```python
from build123d import *

# Parameters (mm, degrees)
F0_W      = 29.9564684167
F0_H      = 51
F0_R      = 5.425
F0_R_2    = 5.95
F1_DEPTH  = 25
F0_W_2    = 18.5217657917
F2_DEPTH  = 25
F0_R_3    = 3.415
F3_DEPTH  = 3.55
F4_R      = 2.34
F5_DEPTH  = 7.5
F7_START  = 14.1
F6_R      = 13
F7_DEPTH  = 10.9
F8_DEPTH  = 10.9
F9_R      = 2.5
F10_DEPTH = 5
F10_TAPER = 15
F11_R     = 5


with BuildPart() as f1:
    # F0 (on Top) → F1 (new body)
    with BuildSketch(Plane.XY):
        with Locations((0, -8)):
            Rectangle(F0_W, F0_H)
        with Locations((0, -25.365)):
            Circle(F0_R, mode=Mode.SUBTRACT)
        Circle(F0_R_2, mode=Mode.SUBTRACT)
    extrude(amount=F1_DEPTH)

    # F0 (on Top) → F2 (join)
    with BuildSketch(Plane.XY):
        with Locations((-24.2391171042, -8)):
            Rectangle(F0_W_2, F0_H)
        with Locations((-25.365, 0)):
            Circle(F0_R, mode=Mode.SUBTRACT)
        with Locations((24.2391171042, -8)):
            Rectangle(F0_W_2, F0_H)
        with Locations((25.365, 0)):
            Circle(F0_R, mode=Mode.SUBTRACT)
    extrude(amount=F2_DEPTH)

    # F0 (on Top) → F3 (join)
    with BuildSketch(Plane.XY):
        with Locations((-25.365, 0)):
            Circle(F0_R)
        with Locations((-25.365, 0)):
            Circle(F0_R_3, mode=Mode.SUBTRACT)
        with Locations((25.365, 0)):
            Circle(F0_R)
        with Locations((25.365, 0)):
            Circle(F0_R_3, mode=Mode.SUBTRACT)
        with Locations((0, -25.365)):
            Circle(F0_R)
        with Locations((0, -25.365)):
            Circle(F0_R_3, mode=Mode.SUBTRACT)
    extrude(amount=F3_DEPTH)

    # F4 (on face) → F5 (cut)
    with BuildSketch(Plane(origin=(0, 17.5, 0), x_dir=(-1, 0, 0), z_dir=(0, 1, 0))):
        with Locations((-10.9382342083, 4.24)):
            Circle(F4_R)
        with Locations((10.9382342083, 4.24)):
            Circle(F4_R)
    extrude(amount=-F5_DEPTH, mode=Mode.SUBTRACT)

    # F6 (on Top) → F7 (cut)
    with BuildSketch(Plane.XY.offset(F7_START)):
        Circle(F6_R)
    extrude(amount=F7_DEPTH, mode=Mode.SUBTRACT)

    # F6 (on Top) → F8 (cut)
    with BuildSketch(Plane.XY):
        Circle(F6_R)
    extrude(amount=F8_DEPTH, mode=Mode.SUBTRACT)

    # F9 (on Top) → F10 (cut)
    with BuildSketch(Plane.XY):
        with Locations((23.62, -23.62)):
            Circle(F9_R)
        with Locations((-23.62, -23.62)):
            Circle(F9_R)
    extrude(amount=F10_DEPTH, taper=F10_TAPER, mode=Mode.SUBTRACT)

    # F11
    f11_edges = [f1.edges().sort_by_distance(p)[0] for p in [
        (33.5, -33.5, 12.5),
        (-33.5, -33.5, 12.5),
        (-33.5, 17.5, 12.5),
        (33.5, 17.5, 12.5),
    ]]
    fillet(f11_edges, radius=F11_R)


solid = f1.part
```
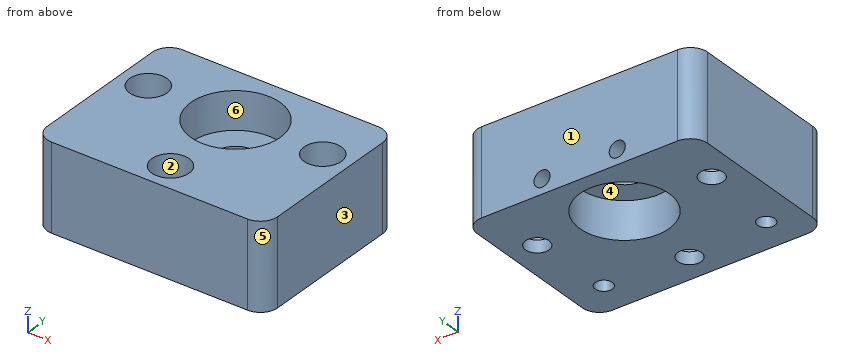
CAD build for the part. Positions are in the model's coordinates, mm. Face numbers are marked on the shaded views. A direction names the side the tool comes from. Coordinates: 2 decimals unless noted, no trailing zeros. Order: outer loops, then holes, each group sorted by start corner. A loop starts at its lowest first (then second) coordinate and runs counter-clockwise, first axis right, second up. Notation, with made-up numbers: (-22, -2) - (6, -2) arc R19 ccw to (6, 17) - close; hole circle Ø11 at (47, 39). An arc over 180 degrees is marked (long way). Answer in a Markdown table with one row per item.
1. Slice it at A-A, the plane y = 0. Give the number of separate pieces and of enclosed holes in the cut face, then the cut area to 3 significant figures.
Answer:
| item | result |
|---|---|
| separate pieces | 4 |
| enclosed holes | 0 |
| area | 556 mm² |
2. Pull direction X, two halves, no side cores. Call the marked faces 1, 2 and 3: +X half, -X half, draft (parallel to the pull), parting line (faces both ways), or undercut.
Answer:
| item | result |
|---|---|
| face 1 | draft |
| face 2 | undercut |
| face 3 | +X half |
3. Flat gauge pins, fed straight in: P1, Ø5, axis at x = 25.5, y = -27.5, coming from the -Z side; P2, Ø8.5, axis at x = 25.5, y = 1, coming from the +Z side; P3, Ø19, axis at x = 0, y = 0, coming from the +Z side; P4, Ø13, axis at x = 2.5, y = 5, coming from the -Z side. Where does each tip first touch, or does it go through?
Answer:
| item | result |
|---|---|
| P1 | z = 0 |
| P2 | z = 3.55 |
| P3 | z = 14.1 |
| P4 | z = 10.9 |
4. Drill centre lines: L1, parallel to Y at x = 0, z = 2; L2, parallel to Y at x = 0, z = 11.6; L3, parallel to X at y = 3.5, z = 11.5. Where is each one in solid material? Low to high. Write a range as from..to.
Answer:
| item | result |
|---|---|
| L1 | -33.5..-28.78, -21.95..-13, 13..17.5 |
| L2 | -33.5..-30.79, -19.94..-5.95, 5.95..17.5 |
| L3 | -33.5..-29.51, -21.22..-4.81, 4.81..21.22, 29.51..33.5 |
5. 3-axis set-ups, long thin cutter, end or side, ignore diameter. For the marked faces 4, 5 and 6: which of +Z, -Z, +X, -X, +Y, -Y reach the whole face in a straight line?
Answer:
| item | result |
|---|---|
| face 4 | -Z |
| face 5 | +Z, -Z, +X, -Y |
| face 6 | +Z |
6. Slice it at D-D, the plane z = 8.5. List the corners of the cut face in (x, y) (3 decimals).
Answer:
| item | result |
|---|---|
| outline | (-33.5, -28.5) arc R5 ccw to (-28.5, -33.5) - (28.5, -33.5) arc R5 ccw to (33.5, -28.5) - (33.5, 12.5) arc R5 ccw to (28.5, 17.5) - (-28.5, 17.5) arc R5 ccw to (-33.5, 12.5) - close; hole circle Ø10.85 at (-25.365, 0); hole circle Ø26 at (0, 0); hole circle Ø10.85 at (0, -25.365); hole circle Ø10.85 at (25.365, 0) |
7. Slice it at B-B, the plane y = -23.62. List the corners of the cut face in (x, z), then the cut area to 3 significant figures.
Answer:
| item | result |
|---|---|
| outline | (-33.5, 0) - (-26.12, 0) - (-24.78, 5) - (-22.46, 5) - (-21.12, 0) - (-2.94, 0) - (-2.94, 3.55) - (-5.14, 3.55) - (-5.14, 25) - (-33.5, 25) - close; (2.94, 0) - (21.12, 0) - (22.46, 5) - (24.78, 5) - (26.12, 0) - (33.5, 0) - (33.5, 25) - (5.14, 25) - (5.14, 3.55) - (2.94, 3.55) - close |
| area | 1,400 mm² |
8. Slice it at C-C, the plane x = 23.62. List the corners of the cut face in (y, z).
Answer:
| item | result |
|---|---|
| outline | (-33.5, 0) - (-26.12, 0) - (-24.78, 5) - (-22.46, 5) - (-21.12, 0) - (-2.94, 0) - (-2.94, 3.55) - (-5.14, 3.55) - (-5.14, 25) - (-33.5, 25) - close; (2.94, 0) - (17.5, 0) - (17.5, 25) - (5.14, 25) - (5.14, 3.55) - (2.94, 3.55) - close |
